The listing builds one solid part. Answer for the finished solid, in the listing's coordinates (mm). Round coordinates to 2 decimals unless told otherwise and drop trailing zeros. Write each loop counter-clockwise with the first axis right and the second up, starting at its lowest first coordinate (ties: lowest second). Pieces come first, ordered by that corner, then holes. Notation, with made-up numbers: (47, 20) -> (83, 20) arc R30 ccw to (83, 59) -> close; hole circle Ø7 at (-37.5, -12.5). An arc over 180 degrees is marked (long way). Write each question's results on one line, items separated by ' | '. Start each with the question number.
```python
from build123d import *

# Parameters (mm, degrees)
F1_DEPTH = 25


# Not quite as in the source:
# - a feature names something its author has since deleted; it is built from what else it names


with BuildPart() as f1:
    # F0 (on Front) → F1 (new body)
    with BuildSketch(Plane.XZ):
        with BuildLine():
            ThreePointArc((5, 40), (4.4370598373, 37.6951138857), (2.875, 35.909232957))
            Line((2.875, 35.909232957), (13.0675283977, 21.406534086))
            ThreePointArc((13.0675283977, 21.406534086), (19.0462821804, 23.222383243), (24.9357240699, 21.1349735599))
            Line((24.9357240699, 21.1349735599), (3.6154854181, 43.4537320671))
            ThreePointArc((3.6154854181, 43.4537320671), (4.6409819592, 41.8604532928), (5, 40))
        make_face()
        with BuildLine():
            ThreePointArc((-9.9215674165, 1.25), (-6.6143782777, 7.5), (0, 10))
            Line((0, 10), (0, 35))
            ThreePointArc((0, 35), (-3.75, 36.6928108612), (-4.9607837082, 40.625))
            Line((-4.9607837082, 40.625), (-9.9215674165, 1.25))
        make_face()
        with BuildLine():
            Line((0, 35), (0, 10))
            ThreePointArc((0, 10), (4.6097722286, 8.8741196746), (8.181534086, 5.75))
            Line((8.181534086, 5.75), (10.6359943118, 7.475))
            ThreePointArc((10.6359943118, 7.475), (8.9664461732, 14.9443542409), (13.0675283977, 21.406534086))
            Line((13.0675283977, 21.406534086), (2.875, 35.909232957))
            ThreePointArc((2.875, 35.909232957), (1.5076744982, 35.2327242992), (0, 35))
        make_face()
        with BuildLine():
            Line((0, 40), (0, 35))
            ThreePointArc((0, 35), (1.5076744982, 35.2327242992), (2.875, 35.909232957))
            Line((2.875, 35.909232957), (0, 40))
        make_face()
        with BuildLine():
            Line((5.75, -8.181534086), (0, 0))
            Line((0, 0), (0, 10))
            ThreePointArc((0, 10), (-6.6143782777, 7.5), (-9.9215674165, 1.25))
            ThreePointArc((-9.9215674165, 1.25), (-5.1564476611, -8.5680247151), (5.75, -8.181534086))
        make_face()
        with BuildLine():
            Line((0, 10), (0, 0))
            Line((0, 0), (8.181534086, 5.75))
            ThreePointArc((8.181534086, 5.75), (4.6097722286, 8.8741196746), (0, 10))
        make_face()
        with BuildLine():
            Line((18.8175283977, 13.225), (24.5675283977, 5.043465914))
            ThreePointArc((24.5675283977, 5.043465914), (27.6916480724, 8.6152277714), (28.8175283977, 13.225))
            ThreePointArc((28.8175283977, 13.225), (28.3520797994, 16.2403489964), (26.9990624837, 18.975))
            Line((26.9990624837, 18.975), (18.8175283977, 13.225))
        make_face()
        with BuildLine():
            ThreePointArc((13.0675283977, 21.406534086), (8.9664461732, 14.9443542409), (10.6359943118, 7.475))
            Line((10.6359943118, 7.475), (18.8175283977, 13.225))
            Line((18.8175283977, 13.225), (13.0675283977, 21.406534086))
        make_face()
        with BuildLine():
            Line((13.0675283977, 21.406534086), (18.8175283977, 13.225))
            Line((18.8175283977, 13.225), (26.9990624837, 18.975))
            Line((26.9990624837, 18.975), (24.9357240699, 21.1349735599))
            ThreePointArc((24.9357240699, 21.1349735599), (19.0462821804, 23.222383243), (13.0675283977, 21.406534086))
        make_face()
        with BuildLine():
            Line((10.6359943118, 7.475), (8.181534086, 5.75))
            ThreePointArc((8.181534086, 5.75), (9.5345514016, 3.0153489964), (10, 0))
            ThreePointArc((10, 0), (8.8741196746, -4.6097722286), (5.75, -8.181534086))
            Line((5.75, -8.181534086), (24.5675283977, 5.043465914))
            ThreePointArc((24.5675283977, 5.043465914), (17.0981741569, 3.3739177755), (10.6359943118, 7.475))
        make_face()
        with BuildLine():
            Line((8.181534086, 5.75), (0, 0))
            Line((0, 0), (5.75, -8.181534086))
            ThreePointArc((5.75, -8.181534086), (8.8741196746, -4.6097722286), (10, 0))
            ThreePointArc((10, 0), (9.5345514016, 3.0153489964), (8.181534086, 5.75))
        make_face()
        with BuildLine():
            Line((18.8175283977, 13.225), (10.6359943118, 7.475))
            ThreePointArc((10.6359943118, 7.475), (17.0981741569, 3.3739177755), (24.5675283977, 5.043465914))
            Line((24.5675283977, 5.043465914), (18.8175283977, 13.225))
        make_face()
        with BuildLine():
            ThreePointArc((-4.9607837082, 40.625), (-3.75, 36.6928108612), (0, 35))
            Line((0, 35), (0, 40))
            Line((0, 40), (2.875, 35.909232957))
            ThreePointArc((2.875, 35.909232957), (4.4370598373, 37.6951138857), (5, 40))
            ThreePointArc((5, 40), (4.6409819592, 41.8604532928), (3.6154854181, 43.4537320671))
            ThreePointArc((3.6154854181, 43.4537320671), (-1.566169898, 44.7483799185), (-4.9607837082, 40.625))
        make_face()
    extrude(amount=F1_DEPTH)


solid = f1.part
```
Q1. The part is cut by section B-B, the plane x = -7. Write down the section's boundary in (y, z), then the cut area to 3 significant figures.
Q2. Find the intervals of material crossed by line 1 (X direction, y = -9.25, z = -1.5); line 2 (Z direction, x = 22, y = -9); line 3 (Z direction, x = 15.5, y = -18.5), in increasing order.
Q3. Each of these flat-tipped pins is pushed along its axis until it touches: pin 1 (8 mm diameter, centred on y = -4.5, z = 26, fed in from -X); pin 2 (1 mm diameter, centred on x = 13, y = -15, fed in from -Z); pin 3 (2 mm diameter, centred on x = 20, y = -16, fed in from +Z). Where does it stop, or does it pass through?
Q4. The part is cut by section A-A, the plane y = -22.75. Write down the section's boundary in (x, z) (3 decimals), then the cut area to 3 significant figures.
Q5. The part is cut by section C-C, the plane z = 2.5. Write down the section's boundary in (x, y).
Answers follow:
1) outline: (-25, -7.14) -> (0, -7.14) -> (0, 24.44) -> (-25, 24.44) -> close | area: 790 mm^2
2) line 1: -9.89 to 15.26 | line 2: 3.24 to 24.21 | line 3: -1.33 to 31.01
3) pin 1: x = -7.31 | pin 2: z = -3.44 | pin 3: z = 27.35
4) outline: (-9.922, 1.25) arc R10 ccw to (5.75, -8.182) -> (24.568, 5.043) arc R10 ccw to (26.999, 18.975) -> (3.615, 43.454) arc R5 ccw to (-4.961, 40.625) -> close | area: 1,370 mm^2
5) outline: (-9.76, -25) -> (20.95, -25) -> (20.95, 0) -> (-9.76, 0) -> close
